Autodesk Inventor part; units mm, degrees
ref_plane "YZ Plane" through (0, 0, 0) normal (1, 0, 0) x (0, 1, 0)
ref_plane "XZ Plane" through (0, 0, 0) normal (0, 1, 0) x (-1, 0, 0)
ref_plane "XY Plane" through (0, 0, 0) normal (0, 0, 1) x (1, 0, 0)
sketch "Sketch1" plane through (0, 0, 0) normal (0, 1, 0) x (-1, 0, 0)
  line L0 (0, 0) -> (50, 0)
  line L1 (50, 0) -> (50, 200)
  line L2 (50, 200) -> (0, 200)
  line L3 (0, 200) -> (0, 0)
  dimension "d1" = 50
  dimension "d2" = 200
extrude "Base" add sketch "Sketch1" along normal blind 4
sketch "Sketch3" plane through (0, 4, 0) normal (0, 1, 0) x (1, 0, 0)
  line L0 (-50, 0) -> (-50, -200)
  line L1 (-50, -200) -> (0, -200)
  line L2 (0, -200) -> (0, 0)
  line L3 (0, 0) -> (-50, 0)
  line L4 (-47, -197) -> (-47, -3)
  line L5 (-47, -3) -> (-3, -3)
  line L6 (-3, -3) -> (-3, -197)
  line L7 (-3, -197) -> (-47, -197)
  line L8 (-25, -198.6939) -> (-25, 11.8917)
  line L9 (-35.2, -200) -> (-14.8, -200)
  line L10 (-14.8, -200) -> (-14.8, -197)
  line L11 (-14.8, -197) -> (-35.2, -197)
  line L12 (-35.2, -197) -> (-35.2, -200)
  point P0 (-25, 0)
  point P1 (-25, -200)
  point P2 (-25, -197)
  dimension "d10" = 3
  dimension "d11" = 20.4
extrude "Muros" add sketch "Sketch3" along normal blind 10.5 contours L3 L8 L5 L4 L7 L12 L1 L0 | L3 L2 L1 L10 L7 L6 L5 L8
sketch "Sketch4" plane through (0, 4, 0) normal (0, 1, 0) x (1, 0, 0)
  line L0 (-35.2, -200) -> (-14.8, -200)
  line L1 (-47, -3) -> (-3, -3)
  line L2 (-28, -200) -> (-22, -200)
  line L3 (-22, -200) -> (-22, -3)
  line L4 (-22, -3) -> (-28, -3)
  line L5 (-28, -3) -> (-28, -200)
  line L6 (-3, -3) -> (-47, -3)
  point P0 (0, 0)
  point P1 (-25, -3)
  point P2 (-25, -3)
  point P3 (-25, -200)
  dimension "d14" = 6
extrude "Rail" cut sketch "Sketch4" against normal blind 2
sketch "Sketch5" plane through (0, 4, 0) normal (0, 1, 0) x (1, 0, 0)
  line L0 (-45.2, -138) -> (-40.2, -138)
  line L1 (-40.2, -138) -> (-40.2, -62)
  line L2 (-40.2, -62) -> (-45.2, -62)
  line L3 (-45.2, -62) -> (-45.2, -138)
  line L4 (-9.8, -138) -> (-4.8, -138)
  line L5 (-4.8, -138) -> (-4.8, -62)
  line L6 (-4.8, -62) -> (-9.8, -62)
  line L7 (-9.8, -62) -> (-9.8, -138)
  line L8 (-28, -200) -> (-28, -3)
  line L9 (-22, -3) -> (-22, -200)
  line L10 (-35.2, -200) -> (-28, -200)
  line L11 (-22, -200) -> (-14.8, -200)
  line L12 (-40.2, -138) -> (-28, -138)
  line L13 (-9.8, -138) -> (-22, -138)
  line L14 (-22, -3) -> (-22, -200)
  line L15 (-40.2, -138) -> (-40.2, -200)
  point P0 (0, 0)
  dimension "d17" = 30.4
  dimension "d18" = 62
  dimension "d19" = 76
  dimension "d20" = 5
extrude "Extrusion4" add sketch "Sketch5" along normal blind 3.2
draft "FaceDraft1" angle 45 pull direction (1, 0, 0) faces at (-43.5333, 5.0667, 138) fixed edges at (-45.2, 5.6, 138)
draft "FaceDraft2" angle 45 pull direction (1, 0, 0) faces at (-41.8667, 5.0667, 62) fixed edges at (-45.2, 5.6, 62)
draft "FaceDraft3" angle 45 pull direction (-1, 0, 0) faces at (-8.1333, 5.0667, 138) fixed edges at (-4.8, 5.6, 138)
draft "FaceDraft4" angle 45 pull direction (-1, 0, 0) faces at (-6.4667, 5.0667, 62) fixed edges at (-4.8, 5.6, 62)
ref_plane "Work Plane1" through (0, 0, 100) normal (0, 0, -1) x (-1, 0, 0)
ref_plane "Work Plane2" through (-25, 0, 200) normal (1, 0, 0) x (0, 0, -1)
sketch "Sketch6" plane through (0, 4, 0) normal (0, 1, 0) x (1, 0, 0)
  line L0 (-45.2, -62) -> (-40.2, -67)
  line L1 (-45.2, -138) -> (-45.2, -62)
  line L2 (-47, -3) -> (-47, -197)
  line L3 (-40.2, -133) -> (-45.2, -138)
  point P0 (0, 0)
  point P1 (-44.8, -59.8)
  point P2 (-44.8, -140.2)
  dimension "d27" = 2.2
  dimension "d28" = 2.2
  dimension "d29" = 2.2
  dimension "d30" = 2.2
hole "Hole1" at (-44.8, 4, 59.8) at (-44.8, 4, 140.2) direction (0, -1, 0) diameter 1 end through all
equation "\"d1\" = base_ancho"
equation "\"d2\" = base_largo"
equation "\"d4\" = base_grosor"
equation "\"d10\" = base_muros_grosor"
equation "\"d11\" = base_muros_separación"
equation "\"d12\" = base_muros_alto"
equation "\"d14\" = base_rail_ancho"
equation "\"d15\" = base_rail_profundidad"
equation "\"d17\" = hoja_ancho + 2 * hoja_diente_ancho + 2 * general_margen"
equation "\"d18\" = -0.5 * base_deslizador_largo + 0.5 * base_largo"
equation "\"d19\" = base_deslizador_largo"
equation "\"d20\" = base_deslizador_ancho"
equation "\"d21\" = base_deslizador_alto"
equation "\"d23\" = base_deslizador_agarre"
equation "\"d24\" = base_deslizador_agarre"
equation "\"d25\" = base_deslizador_agarre"
equation "\"d26\" = base_deslizador_agarre"
equation "\"d31\" = traba_eje_diametro"
properties part number "Base"
Part model, mm, in its own coordinate system. A direction names the side the tool comes from. Round coordinates to 2 decimals unless told otherwise and drop trailing zeros. Write each loop counter-clockwise with the first axis right and the second up, starting at its lowest first coordinate (ties: lowest second). Pieces come first, ordered by that corner, then holes.
Item 1: Cut at A-A, the plane z = 86.5. Give the cut face in (x, y).
Results:
outline: (-50, 0) - (0, 0) - (0, 14.5) - (-3, 14.5) - (-3, 4) - (-4.8, 4) - (-4.8, 7.2) - (-9.8, 7.2) - (-9.8, 4) - (-22, 4) - (-22, 2) - (-28, 2) - (-28, 4) - (-40.2, 4) - (-40.2, 7.2) - (-45.2, 7.2) - (-45.2, 4) - (-47, 4) - (-47, 14.5) - (-50, 14.5) - close
Item 2: Probe L1, parallel to X at y = 3, z = 140.2; L2, parallel to Z at x = -44.8, y = 1.5; L3, parallel to X at y = 4.5, z = 87. List the from-to ranges inside material, lowest first.
Results:
L1: x = -50 to -45.3, -44.3 to -28, -22 to 0
L2: z = 0 to 59.3, 60.3 to 139.7, 140.7 to 200
L3: x = -50 to -47, -45.2 to -40.2, -9.8 to -4.8, -3 to 0
Item 3: Cut at C-C, the plane x = -20. Give the cut face in (y, z).
Results:
outline: (0, 0) - (14.5, 0) - (14.5, 3) - (4, 3) - (4, 200) - (0, 200) - close
Item 4: Cut at B-B, the plane y = 10.5. Give the cut face in (x, z), plus the area to 3 significant figures.
Results:
outline: (-50, 0) - (0, 0) - (0, 200) - (-14.8, 200) - (-14.8, 197) - (-3, 197) - (-3, 3) - (-47, 3) - (-47, 197) - (-35.2, 197) - (-35.2, 200) - (-50, 200) - close
area: 1,400 mm2
Item 5: Two-plate mould, pull along X, no slides. Class faces 1 (the flat face through (-50, 7, 99)), 2 (the flat face through (-40.2, 6, 100)), 3 (the flat face through (0, 7, 101)): +X half, -X half, draft (parallel to the pull), parting line (faces both ways), or undercut.
Results:
face 1: -X half
face 2: undercut
face 3: +X half
Item 6: Which spindle directions (+Z, -Z, +X, -X, +Y, -Y) get a long thin tool onto all of the face, cutting with end or side? Do faces 4 (the flat face through (-7.3, 5.6, 135.5)), 5 (the flat face through (-47.3, 14.5, 99.5)). Say none if no direction does.
Results:
face 4: +Y
face 5: +Z, -Z, +X, -X, +Y
Item 7: Drop flat-ended pins along their axis: pin 1 Ø2.5 at (x, z) = (-42, 102.5) entering from +Y; pin 2 Ø6.5 at (x, z) = (-25.5, 110) entering from +Y. Give the stop position or say it passes through.
Results:
pin 1: stops at y = 7.2
pin 2: stops at y = 4
Item 8: Cut at D-D, the plane z = 171. Give the cut face in (x, y), plus the area to 3 significant figures.
Results:
outline: (-50, 0) - (0, 0) - (0, 14.5) - (-3, 14.5) - (-3, 4) - (-22, 4) - (-22, 2) - (-28, 2) - (-28, 4) - (-47, 4) - (-47, 14.5) - (-50, 14.5) - close
area: 251 mm2
